from build123d import *

# Parameters (mm, degrees)
F0_W     = 17.543719
F0_H     = 9.835118
F1_DEPTH = 25.4


with BuildPart() as f1:
    # F0 (on Front) → F1 (new body)
    with BuildSketch(Plane.XZ):
        Polygon((-26.578831, 2.592185), (-26.578831, 0), (11.033846, 0), (11.033846, 2.592185), (-23.654874, 2.592185), align=None)
        Polygon((-23.654874, 6.446487), (-23.654874, 2.592185), (11.033846, 2.592185), (11.033846, 6.446487), (-18.737316, 6.446487), align=None)
        Polygon((-18.737316, 6.446487), (11.033846, 6.446487), (11.033846, 11.231139), (-12.091967, 11.231139), (-18.737316, 11.231139), align=None)
        Polygon((-12.091967, 11.231139), (11.033846, 11.231139), (11.033846, 18.806836), (-6.509873, 18.806836), (-12.091967, 18.806836), align=None)
        with Locations((2.261986, 23.724395)):
            Rectangle(F0_W, F0_H)
    extrude(amount=F1_DEPTH)


solid = f1.part
Verification items for the finished model (mm, model axes). A direction names the side the tool comes from. Give positions to 0.01 mm unless a question says otherwise; leave off trailing zeros. Write each loop counter-clockwise with the first axis right and the second up, starting at its lowest first coordinate (ties: lowest second). Pieces come first, ordered by that corner, then holes.
(1) Cross-section at C-C (x = -21). Enter the section's corners in (y, z), plus the area to 3 significant figures.
(2) Gauge pin test, flat ends, axial feed: pin 1 (3 mm diameter, centred on x = -25, y = -16, fed in from +Z); pin 2 (12 mm diameter, centred on y = -7, z = 20, fed in from -X); pin 3 (5.5 mm diameter, centred on x = -20, y = -11.5, fed in from +Z). Record the tip position at first contact, or that the pin passes through.
(3) Cross-section at A-A (y = -20.5). Enter the section's corners in (x, z).
(4) Cross-section at B-B (z = 10). Enter the section's corners in (x, y), plus the area to 3 significant figures.
(5) Access from +Z, -Z, +X, -X, +Y, -Y to the whole of each face (thin tool, end or side, straight path). Record for faces 1 (the face through (11.034, -13, 9)), 2 (the face through (-9, -13, 18.807)).
(6) Material ranges on line 1 (Z direction, x = -22.5, y = -10.5); line 2 (Z direction, x = -8, y = -7.75); line 3 (X direction, y = -2, z = 5.75), recorded low to high.
Worked out:
1. outline: (-25.4, 0) - (0, 0) - (0, 6.45) - (-25.4, 6.45) - close
1. area: 164 mm2
2. pin 1: stops at z = 6.45
2. pin 2: stops at x = -12.09
2. pin 3: stops at z = 11.23
3. outline: (-26.58, 0) - (11.03, 0) - (11.03, 28.64) - (-6.51, 28.64) - (-6.51, 18.81) - (-12.09, 18.81) - (-12.09, 11.23) - (-18.74, 11.23) - (-18.74, 6.45) - (-23.65, 6.45) - (-23.65, 2.59) - (-26.58, 2.59) - close
4. outline: (-18.74, -25.4) - (11.03, -25.4) - (11.03, 0) - (-18.74, 0) - close
4. area: 756 mm2
5. face 1: +Z, -Z, +X, +Y, -Y
5. face 2: +Z, -X, +Y, -Y
6. line 1: z = 0 to 6.45
6. line 2: z = 0 to 18.81
6. line 3: x = -23.65 to 11.03
